Autodesk Inventor part; units mm, degrees
ref_plane "cp_XY" through (0, 0, 0) normal (0, -1, 0) x (1, 0, 0)
ref_plane "cp_YZ" through (0, 0, 0) normal (1, 0, 0) x (0, 0, 1)
ref_plane "cp_ZX" through (0, 0, 0) normal (0, 0, 1) x (0, -1, 0)
sketch "Sketch_1" plane through (0, 0, 0) normal (0, 1, 0) x (-1, 0, 0)
  arc A0 (0, -5) -> (-4.7697, -1.5) centre (0, 0) ccw
  line L0 (-4.7697, -1.5) -> (-17, -1.5)
  arc A1 (-17, -1.5) -> (-18, -2.5) centre (-17, -2.5) ccw
  line L1 (-18, -2.5) -> (-18, -5)
  line L2 (-18, -5) -> (0, -5)
  circle A2 centre (0, 0) radius 2.5
extrude "Extrusion1" add sketch "Sketch_1" along normal mid plane 47
sketch "Sketch_2" plane through (0, 0, 0) normal (0, 0, 1) x (1, 0, 0)
  line L0 (-10, -23.5) -> (5.5, -23.5)
  line L1 (5.5, -23.5) -> (5.5, -11.25)
  line L2 (5.5, -11.25) -> (-5, -11.25)
  line L3 (-5, -11.25) -> (-5, -0.5)
  line L4 (-5, -0.5) -> (5.5, -0.5)
  line L5 (5.5, -0.5) -> (5.5, 12.25)
  line L6 (5.5, 12.25) -> (-5, 12.25)
  line L7 (-5, 12.25) -> (-5, 23.5)
  line L8 (-5, 23.5) -> (-10, 23.5)
  line L9 (-10, 23.5) -> (-10, -23.5)
extrude "Extrusion2" cut sketch "Sketch_2" along normal mid plane 10
sketch "Sketch_4" plane through (10.5, 0, 0) normal (1, 0, 0) x (0, 0, -1)
  line L0 (5, 12.5) -> (1.5, 12.5)
  line L1 (1.5, 12.5) -> (1.5, 18)
  line L2 (1.5, 18) -> (4.25, 15.25)
  line L3 (4.25, 15.25) -> (5, 15.25)
  line L4 (5, 15.25) -> (5, 12.5)
  line L5 (5, 12.5) -> (1.5, 12.5)
revolve "Revolution1" cut sketch "Sketch_4" angle 360 about axis through (10.5, 12.5, -5) along (0, 0, -1)
sketch "Sketch_5" plane through (10.5, 0, 0) normal (1, 0, 0) x (0, 0, -1)
  line L0 (5, -12.5) -> (1.5, -12.5)
  line L1 (1.5, -12.5) -> (1.5, -7)
  line L2 (1.5, -7) -> (4.25, -9.75)
  line L3 (4.25, -9.75) -> (5, -9.75)
  line L4 (5, -9.75) -> (5, -12.5)
  line L5 (5, -12.5) -> (1.5, -12.5)
revolve "Revolution2" cut sketch "Sketch_5" angle 360 about axis through (10.5, -12.5, -5) along (0, 0, -1)
sketch "Sketch_10" plane through (0, 0, 0) normal (0, 0, 1) x (1, 0, 0)
  line L0 (0, 23.5) -> (0, 25.2)
  line L1 (2.5, 23.5) -> (4.5, 23.5)
  line L2 (4.5, 23.5) -> (4.5, 24.5)
  line L3 (4.5, 24.5) -> (4, 24.5)
  line L4 (4, 24.5) -> (4, 25.2)
  line L5 (4, 25.2) -> (2.5, 25.2)
  line L6 (2.5, 25.2) -> (2.5, 23.5)
revolve "Revolution3" add sketch "Sketch_10" angle 360 about axis through (0, 23.5, 0) along (0, -1, 0)
ref_plane "cp_XY" through (0, 0, 0) normal (0, -1, 0) x (1, 0, 0)
ref_plane "cp_YZ" through (0, 0, 0) normal (1, 0, 0) x (0, 0, 1)
ref_plane "cp_ZX" through (0, 0, 0) normal (0, 0, 1) x (0, -1, 0)
ref_plane "bolt1_XY" through (10.5, 12.5, -4.25) normal (0, 0, 1) x (1, 0, 0)
ref_plane "bolt1_YZ" through (10.5, 12.5, -4.25) normal (1, 0, 0) x (0, 1, 0)
ref_plane "bolt1_ZX" through (10.5, 12.5, -4.25) normal (0, 1, 0) x (0, 0, 1)
ref_plane "bolt2_XY" through (10.5, -12.5, -4.25) normal (0, 0, 1) x (1, 0, 0)
ref_plane "bolt2_YZ" through (10.5, -12.5, -4.25) normal (1, 0, 0) x (0, 1, 0)
ref_plane "bolt2_ZX" through (10.5, -12.5, -4.25) normal (0, 1, 0) x (0, 0, 1)
ref_plane "nut1_XY" through (10.5, 12.5, -5) normal (0, 0, 1) x (1, 0, 0)
ref_plane "nut1_YZ" through (10.5, 12.5, -5) normal (1, 0, 0) x (0, 1, 0)
ref_plane "nut1_ZX" through (10.5, 12.5, -5) normal (0, 1, 0) x (0, 0, 1)
ref_plane "nut2_XY" through (10.5, -12.5, -5) normal (0, 0, 1) x (1, 0, 0)
ref_plane "nut2_YZ" through (10.5, -12.5, -5) normal (1, 0, 0) x (0, 1, 0)
ref_plane "nut2_ZX" through (10.5, -12.5, -5) normal (0, 1, 0) x (0, 0, 1)
properties part number "HHPMGS5p2"
Read the model definition and answer for the solid it produces. Units are mm, in the model's axes. A direction names the side the tool comes from. Coordinates: 2 decimals unless noted, no trailing zeros. Loops run counter-clockwise (first coordinate to the right, second up) from the corner with the lowest first, then second, coordinate; pieces in that order, holes last. Notation, with made-up numbers: (24.5, 6) - (65.5, 6) arc R11 cw to (65.5, 16) - close; hole circle Ø7 at (23.5, 12). An arc over 180 degrees is marked (long way). Answer in a Markdown table with one row per item.
1. Straight lines are drawn through the part: line 1 (X direction, y = 15, z = 0); line 2 (Y direction, x = -1.5, z = -4); line 3 (Y direction, x = -3, z = 1.25). For each, find the intervals that lie inside material, in ascending order.
Conclusion:
| item | result |
|---|---|
| line 1 | x = -5 to -2.5, 2.5 to 5 |
| line 2 | y = -11.25 to -0.5, 12.25 to 24.5 |
| line 3 | y = -11.25 to -0.5, 12.25 to 25.2 |
2. Find section D-D, the plane x = -3.5. Write down the section's boundary in (y, z), then the cut area to 3 significant figures.
Conclusion:
| item | result |
|---|---|
| outline | (-11.25, -3.57) - (-0.5, -3.57) - (-0.5, 3.57) - (-11.25, 3.57) - close; (12.25, -3.57) - (23.5, -3.57) - (23.5, -2.83) - (24.5, -2.83) - (24.5, -1.94) - (25.2, -1.94) - (25.2, 1.94) - (24.5, 1.94) - (24.5, 2.83) - (23.5, 2.83) - (23.5, 3.57) - (12.25, 3.57) - close |
| area | 165 mm² |
3. Determine the mould class of faces 1 (the face through (-0.59, 24.01, -4.46)), 2 (the face through (11, 0, -5)), 3 (the face through (18, 0, -4)), 4 (the face through (13.09, 13.85, -4.08)) for opening direction X: +X half, -X half, draft (parallel to the pull), parting line (faces both ways), or undercut.
Conclusion:
| item | result |
|---|---|
| face 1 | parting line |
| face 2 | draft |
| face 3 | +X half |
| face 4 | undercut |
4. Given pin 1 (9 mm diameter, centred on x = 10.5, y = 12.5, fed in from +Z); pin 2 (2 mm diameter, centred on x = -2.5, y = -6, fed in from -Z); pin 3 (4 mm diameter, centred on x = 10, y = 3, fed in from +Z), each flat-ended and moving along its own axis, determine where each tip first touches the part or whether it passes through.
Conclusion:
| item | result |
|---|---|
| pin 1 | stops at z = -2.5 |
| pin 2 | stops at z = -4.77 |
| pin 3 | stops at z = -1.5 |
5. Which of the six approach directions +Z, -Z, +X, -X, +Y, -Y give full straight-line access (tool end or side, diameter ignored) to faces 5 (the face through (2, 25.2, 2)), 6 (the face through (-3, 24.5, -3)), 7 (the face through (5.5, -17, -3)), 8 (the face through (1.5, 12.25, -2.3))?
Conclusion:
| item | result |
|---|---|
| face 5 | +Z, -Z, +X, -X, +Y |
| face 6 | +Y |
| face 7 | +Z, -Z, -X, -Y |
| face 8 | +Z, -Z, -X |
6. Find section C-C, the plane y = -3. Write down the section's boundary in (x, z).
Conclusion:
| item | result |
|---|---|
| outline | (0, -5) - (18, -5) - (18, -2.5) arc R1 ccw to (17, -1.5) - (4.77, -1.5) arc R5 ccw (long way) to start; hole circle Ø5 at (0, 0) |
7. Find section A-A, the plane x = 10.5. Write down the section's boundary in (y, z), then the cut area to 3 significant figures.
Conclusion:
| item | result |
|---|---|
| outline | (-23.5, -5) - (-15.25, -5) - (-15.25, -4.25) - (-18, -1.5) - (-23.5, -1.5) - close; (-9.75, -5) - (9.75, -5) - (9.75, -4.25) - (7, -1.5) - (-7, -1.5) - (-9.75, -4.25) - close; (15.25, -5) - (23.5, -5) - (23.5, -1.5) - (18, -1.5) - (15.25, -4.25) - close |
| area | 111 mm² |
8. Find section B-B, the plane z = 3. Write down the section's boundary in (x, y), then the cut area to 3 significant figures.
Conclusion:
| item | result |
|---|---|
| outline | (-4, -11.25) - (4, -11.25) - (4, -0.5) - (-4, -0.5) - close; (-4, 12.25) - (4, 12.25) - (4, 23.5) - (3.35, 23.5) - (3.35, 24.5) - (2.65, 24.5) - (2.65, 25.2) - (-2.65, 25.2) - (-2.65, 24.5) - (-3.35, 24.5) - (-3.35, 23.5) - (-4, 23.5) - close |
| area | 186 mm² |
